```python
from build123d import *

# Parameters (mm, degrees)
SKETCH1_R           = 20.4
SKETCH1_R_2         = 14.725
BOSS_EXTRUDE1_DEPTH = 34.3
FILLET1_R           = 8
FILLET2_R           = 5.4
CUT_EXTRUDE1_DEPTH  = 90.29876936
CIRPATTERN1_COUNT   = 8
FILLET3_R           = 10
CHAMFER1_SIZE       = 1
FILLET4_R           = 2


with BuildPart() as part:
    # Sketch1 → Boss-Extrude1 (new body)
    with BuildSketch(Plane.XY):
        Circle(SKETCH1_R)
        Circle(SKETCH1_R_2, mode=Mode.SUBTRACT)
    extrude(amount=BOSS_EXTRUDE1_DEPTH)

    # Sketch3 → Revolve1 (revolve)
    with BuildSketch(Plane(origin=(0, 0, 0), x_dir=(1, 0, 0), z_dir=(0, 1, 0)), mode=Mode.PRIVATE) as revolve1_sk:
        Polygon((-20.4, 0), (-58.3, -12.314456487), (-58.3, -23.814456487), (-55.7, -23.814456487), (-55.7, -14.20346706), (-20.4, -2.733801783), align=None)
    revolve(revolve1_sk.sketch.rotate(Axis((0, 0, 0), (0, 0, -1)), 180), axis=Axis((0, 0, 0), (0, 0, -1)))

    # Fillet1
    fillet1_edges = [part.edges().sort_by_distance(p)[0] for p in [
        (-58.3, 0, 12.314456487),
    ]]
    fillet(fillet1_edges, radius=FILLET1_R)

    # Fillet2
    fillet2_edges = [part.edges().sort_by_distance(p)[0] for p in [
        (-55.7, 0, 14.20346706),
    ]]
    fillet(fillet2_edges, radius=FILLET2_R)

    # Sketch4 → Cut-Extrude1 (cut, through all)
    with BuildSketch(Plane(origin=(0, 0, 0), x_dir=(-1, 0, 0), z_dir=(0, 0, -1))):
        with BuildLine():
            Line((-3.35, 14.338867633), (-3.35, 16.998032974))
            ThreePointArc((-3.35, 16.998032974), (0, 17.325), (3.35, 16.998032974))
            Line((3.35, 16.998032974), (3.35, 14.338867633))
            ThreePointArc((3.35, 14.338867633), (0, 14.725), (-3.35, 14.338867633))
        make_face()
    cut_extrude1 = extrude(amount=-CUT_EXTRUDE1_DEPTH, mode=Mode.SUBTRACT)

    # CirPattern1: Cut-Extrude1 ×8 about axis
    cirpattern1_axis = Axis((0, 0, 0), (0, 0, 1))
    for i in range(1, CIRPATTERN1_COUNT):
        add(cut_extrude1.rotate(cirpattern1_axis, i * 360 / CIRPATTERN1_COUNT), mode=Mode.SUBTRACT)

    # Fillet3
    fillet3_edges = [part.edges().sort_by_distance(p)[0] for p in [
        (-20.4, 0, 0),
    ]]
    fillet(fillet3_edges, radius=FILLET3_R)

    # Sketch5 → Cut-Revolve1 (revolve, cut)
    with BuildSketch(Plane(origin=(0, 0, 0), x_dir=(1, 0, 0), z_dir=(0, 1, 0))):
        Polygon((-17.325, -34.3), (-17.325, -33.8), (-13.825, -30.3), (-13.825, -34.3), align=None)
        Polygon((-17.825, -34.3), (-17.325, -33.8), (-17.325, -34.3), align=None)
    revolve(axis=Axis((0, 0, 0), (0, 0, -1)), mode=Mode.SUBTRACT)

    # Chamfer1
    chamfer1_edges = [part.edges().sort_by_distance(p)[0] for p in [
        (-13.604126116, -5.635013542, 0),
        (-13.604126116, 5.635013542, 0),
        (-5.635013542, 13.604126116, 0),
        (5.635013542, 13.604126116, 0),
        (13.604126116, 5.635013542, 0),
        (13.604126116, -5.635013542, 0),
        (5.635013542, -13.604126116, 0),
        (-5.635013542, -13.604126116, 0),
    ]]
    chamfer(chamfer1_edges, length=CHAMFER1_SIZE)

    # Fillet4
    fillet4_edges = [part.edges().sort_by_distance(p)[0] for p in [
        (-20.4, 0, 2.733801783),
    ]]
    fillet(fillet4_edges, radius=FILLET4_R)


solid = part.part
```
The model under review builds one solid part; all positions refer to its coordinate system, in mm. A direction names the side the tool comes from. Round coordinates to 2 decimals unless told otherwise and drop trailing zeros.
Item 1: For faces 4 (the face through (-14.07, 5.79, 0.51)), 5 (the face through (9.41, -18.1, 19.69)), 6 (the face through (0.047, 17.325, 16.663)), list the 3-axis set-ups (+Z, -Z, +X, -X, +Y, -Y) from which the entire face can be reached by the end or side of a thin tool; tool diameter is ignored.
Determined:
face 4: -Z
face 5: +Z
face 6: +Z, -Z
Item 2: Mouldability with a two-part tool opening along Y and no side actions: class faces 1 (the face through (-5.6, 13.62, 15.89)), 2 (the face through (-5.79, -14.07, 0.51)), 3 (the face through (30, 47.2, 23.814)) as released by +Y, released by -Y, zero draft, split by the parting line, or undercut.
Determined:
face 1: undercut
face 2: undercut
face 3: zero draft
Item 3: For line 1 (Y direction, x = 0, z = 20) (3 decimals); line 2 (X direction, y = 13, z = 28); line 3 (Z direction, x = 28, y = -18.5), list the stretches that pass through material, from the lowest coordinate up.
Determined:
line 1: y = -58.3 to -55.7, -20.4 to -17.325, 17.325 to 20.4, 55.7 to 58.3
line 2: x = -15.72 to -11.45, -8.26 to -6.92, 6.92 to 8.26, 11.45 to 15.72
line 3: z = 4.28 to 7.01
Item 4: Clearance check with flat-ended pins moving along their axes: pin 1 Ø3 at (y, z) = (15, 18.5) entering from -X; pin 2 Ø0.8 at (y, z) = (16, 22.5) entering from +X; pin 3 Ø0.8 at (x, z) = (-15.5, 12.5) entering from -Y; pin 4 Ø4 at (x, z) = (-32.5, 27.5) entering from +Y. State where each tip first meets the part, or that it passes through.
Determined:
pin 1: stops at x = -56.72
pin 2: stops at x = 56.17
pin 3: stops at y = -54.2
pin 4: passes through
